Input: dimensioned drawing with shaded views. Units: mm. Origin: part minimum x, y, z. Give positions to 0.01 mm unless a question says otherwise; leave off trailing zeros. Write each loop counter-clockwise with the first axis right and the second up, starting at its lowest first coordinate (ties: lowest second). Pieces come first, ordered by that corner, then holes. Notation, with made-up numbers: M 62,29.25 L 76,29.25 A20 ccw 76,36.25 Z; hole C 25.25,26.25 d6. An arc over 180 degrees is marked long. Answer as a JSON object with one key per item and string values.
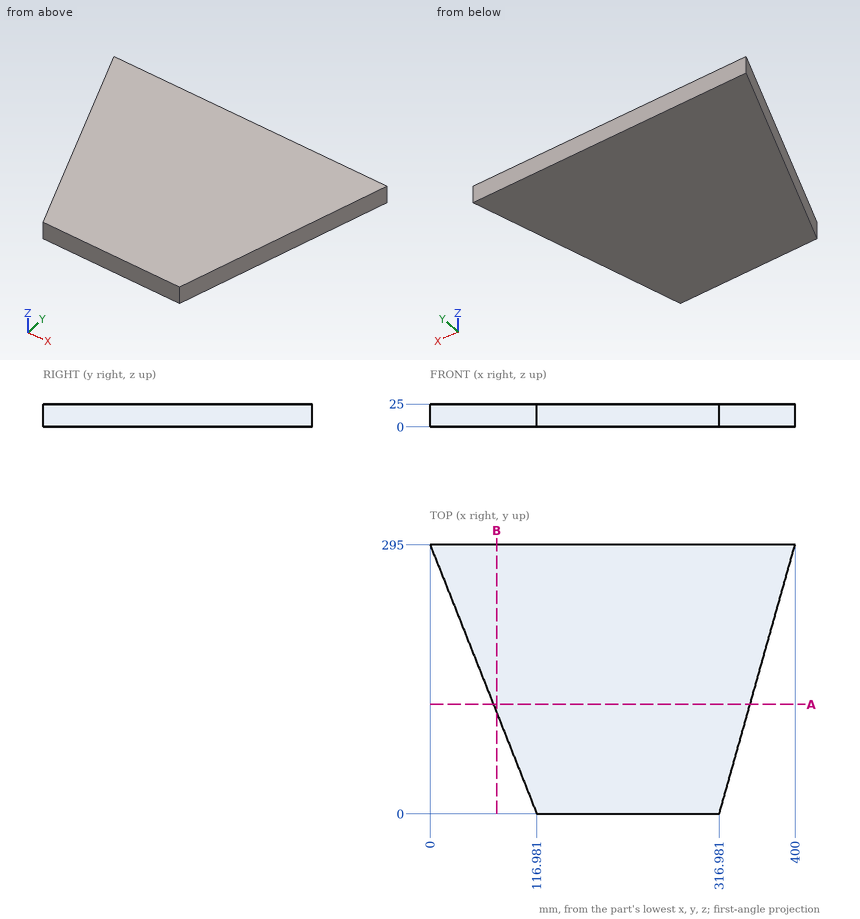
1) Cut plane B-B on x = 73. Return loops of the section in (y, z), and give its area (3 significant figures).
Geometry check:
{"outline": "M 110.91,0 L 295,0 L 295,25 L 110.91,25 Z", "area": "4,600 mm2"}
2) Line query: line 1 (X direction, y = 206, z = 8.75); line 2 (X direction, y = 89.5, z = 13.25). Output: solid intervals per line, ascending. Write a range as from..to.
Geometry check:
{"line 1": "x = 35.29..374.95", "line 2": "x = 81.49..342.17"}
3) Cut plane A-A on y = 120. Return loops of the section in (x, z), and give its area (3 significant figures).
Geometry check:
{"outline": "M 69.4,0 L 350.75,0 L 350.75,25 L 69.4,25 Z", "area": "7,030 mm2"}
4) Contact query for flat-ended pins moving along their axis: P1, Ø2, axis at y = 168.5, z = 19.5, coming from the -X side; P2, Ø2, axis at y = 187.5, z = 6.5, coming from the +X side; P3, Ø4, axis at y = 103, z = 3.5, coming from the +X side. Output: stop coordinate, or through.
Geometry check:
{"P1": "stops at x = 49.77", "P2": "stops at x = 370.03", "P3": "stops at x = 346.53"}
